Here's how the part is built. I have some questions about the finished solid (model axes, mm). Coordinates: 2 decimals unless noted, no trailing zeros. Loops run counter-clockwise (first coordinate to the right, second up) from the corner with the lowest first, then second, coordinate; pieces in that order, holes last. Notation, with made-up numbers: (22, 23.25) - (80, 23.25) arc R23 ccw to (80, 32.25) - close; hole circle Ø11 at (11.25, 9). An arc over 180 degrees is marked (long way). Use a Markdown table: item, result.
```python
from build123d import *

# Parameters (mm, degrees)
SKETCH1_R           = 22.5
BOSS_EXTRUDE1_DEPTH = 3
BOSS_EXTRUDE2_START = 37
SKETCH2_R           = 22.5
SKETCH2_R_2         = 18
BOSS_EXTRUDE2_DEPTH = 37
FILLET1_R           = 5
BOSS_EXTRUDE3_START = -6
SKETCH3_R           = 18
SKETCH3_R_2         = 17.100000000000033
BOSS_EXTRUDE3_DEPTH = 6


with BuildPart() as part:
    # Sketch1 → Boss-Extrude1 (new body)
    with BuildSketch(Plane(origin=(0, 0, 0), x_dir=(1, 0, 0), z_dir=(0, 1, 0))):
        with Locations(Location((0, 0, 0), (0, 0, 270))):
            Circle(SKETCH1_R)
    extrude(amount=BOSS_EXTRUDE1_DEPTH)

    # Sketch2 → Boss-Extrude2 (add)
    with BuildSketch(Plane(origin=(0, 0, 0), x_dir=(-1, 0, 0), z_dir=(0, -1, 0)).offset(BOSS_EXTRUDE2_START)):
        with Locations(Location((0, 0, 0), (0, 0, 90))):
            Circle(SKETCH2_R)
        with Locations(Location((0, 0, 0), (0, 0, 90))):
            Circle(SKETCH2_R_2, mode=Mode.SUBTRACT)
    extrude(amount=-BOSS_EXTRUDE2_DEPTH)

    # Fillet1
    # the kernel refuses this fillet: 5 mm, written as the material it takes off along each edge
    with BuildSketch(Plane(origin=(0, -37, 0), x_dir=(-6e-17, 0, -1), z_dir=(-1, 0, 6e-17))) as fillet1_piece_1:
        with BuildLine():
            CenterArc((23, -4.974937185533101), FILLET1_R, 95.73917047726678, 84.26082952273322)
            Line((18, -4.974937185533101), (17.9, -4.974937185533101))
            Line((17.9, -4.974937185533101), (17.9, 0))
            Line((17.9, 0), (18, 0.10000000000000142))
            ThreePointArc((18, 0.10000000000000142), (20.25, 0.10000000000000142), (22.49, 0.09949874371066159))
            Line((22.49, 0.09949874371066159), (22.5, 0))
        make_face()
    revolve(axis=Axis((0, -37, 0), (0, -1, 0)), mode=Mode.SUBTRACT)

    # Sketch3 → Boss-Extrude3 (add)
    with BuildSketch(Plane(origin=(0, 3, 0), x_dir=(1, 0, 0), z_dir=(0, 1, 0)).offset(BOSS_EXTRUDE3_START)):
        with Locations(Location((0, 0, 0), (0, 0, 270))):
            Circle(SKETCH3_R)
        with Locations(Location((0, 0, 0), (0, 0, 270))):
            Circle(SKETCH3_R_2, mode=Mode.SUBTRACT)
    extrude(amount=BOSS_EXTRUDE3_DEPTH)


solid = part.part
```
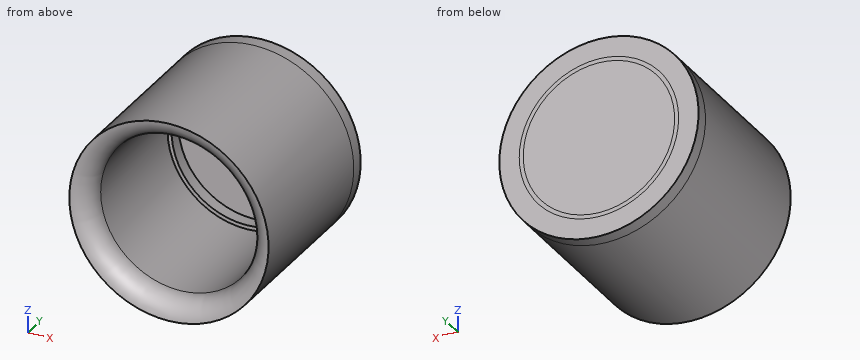
Q1. I want a section at B-B, the plane y = -10. Write out the boundary of the cut face in (x, z).
Check values:
| item | result |
|---|---|
| outline | circle Ø45 at (0, 0); hole circle Ø36 at (0, 0) |
Q2. I want a section at C-C, the plane z = 0. Write out the boundary of the cut face in (x, y), then the cut area to 3 significant figures.
Check values:
| item | result |
|---|---|
| outline | (-22.5, -37) arc R5 ccw to (-18, -32.03) - (-18, -3) - (-17.1, -3) - (-17.1, 0) - (17.1, 0) - (17.1, -3) - (18, -3) - (18, -32.03) arc R5 ccw to (22.5, -37) - (22.5, 3) - (-22.5, 3) - close |
| area | 463 mm^2 |
Q3. I want a section at A-A, the plane x = 0. Write out the boundary of the cut face in (y, z).
Check values:
| item | result |
|---|---|
| outline | (-37, -22.5) - (3, -22.5) - (3, 22.5) - (-37, 22.5) arc R5 ccw to (-32.03, 18) - (-3, 18) - (-3, 17.1) - (0, 17.1) - (0, -17.1) - (-3, -17.1) - (-3, -18) - (-32.03, -18) arc R5 ccw to start |
Q4. Will these pins go through, and if not, where does the flat tip stop? P1, Ø8, axis at x = -18, y = -11.5, coming from the +Z side; P2, Ø1, axis at y = -19.5, z = -12, coming from the +X side; P3, Ø18, axis at x = 3.5, z = 2.5, coming from the -Y side.
Check values:
| item | result |
|---|---|
| P1 | z = 17.61 |
| P2 | x = 19.34 |
| P3 | y = 0 |
Q5. Please list where these lines run through material, in increasing order: L1, parallel to Z at x = 0, y = -0.8; L2, parallel to X at y = -13.5, z = 0. Write a range as from..to.
Check values:
| item | result |
|---|---|
| L1 | -22.5..-17.1, 17.1..22.5 |
| L2 | -22.5..-18, 18..22.5 |
